Design review of the part shown in the three views and the two pictorial views. Dimensions are in mm from the part's minimum x, y and z. A direction names the side the tool comes from. Round coordinates to 2 decimals unless told otherwise and drop trailing zeros. Loops run counter-clockwise (first coordinate to the right, second up) from the corner with the lowest first, then second, coordinate; pieces in that order, holes last.
1. Consider section B-B on z = 15. State the section outline as (x, y) points.
2. Consider section D-D on y = 23. State the section outline as (x, z) points, then the cut area to 3 significant figures.
3. Tool access review of the marked faces 1 and 2: name each direction out of +Z, -Z, +X, -X, +Y, -Y from which nothing blocks a thin tool from reaching the whole face with its end or side.
4. Clearance check with flat-ended pins moving along their axes: pin 1 Ø10 at (x, z) = (15.5, 9.5) entering from -Y; pin 2 Ø10 at (y, z) = (31.5, 36) entering from +X; pin 3 Ø0.6 at (x, z) = (32.5, 0.5) entering from +Y; pin 4 Ø1 at (x, y) = (26, 0.5) entering from -Z. State where each tip first meets the part, or that it passes through.
5. Consider section C-C on y = 14. State the section outline as (x, z) points.
6. To check wall thickness, follow line 1 along Y through (x, z) = (31.5, 31.5); line 2 along Z through (x, y) = (20, 17); line 3 along X through (y, z) = (41.5, 30.5). State the ranges of each line that lie inside material, in increasing order.
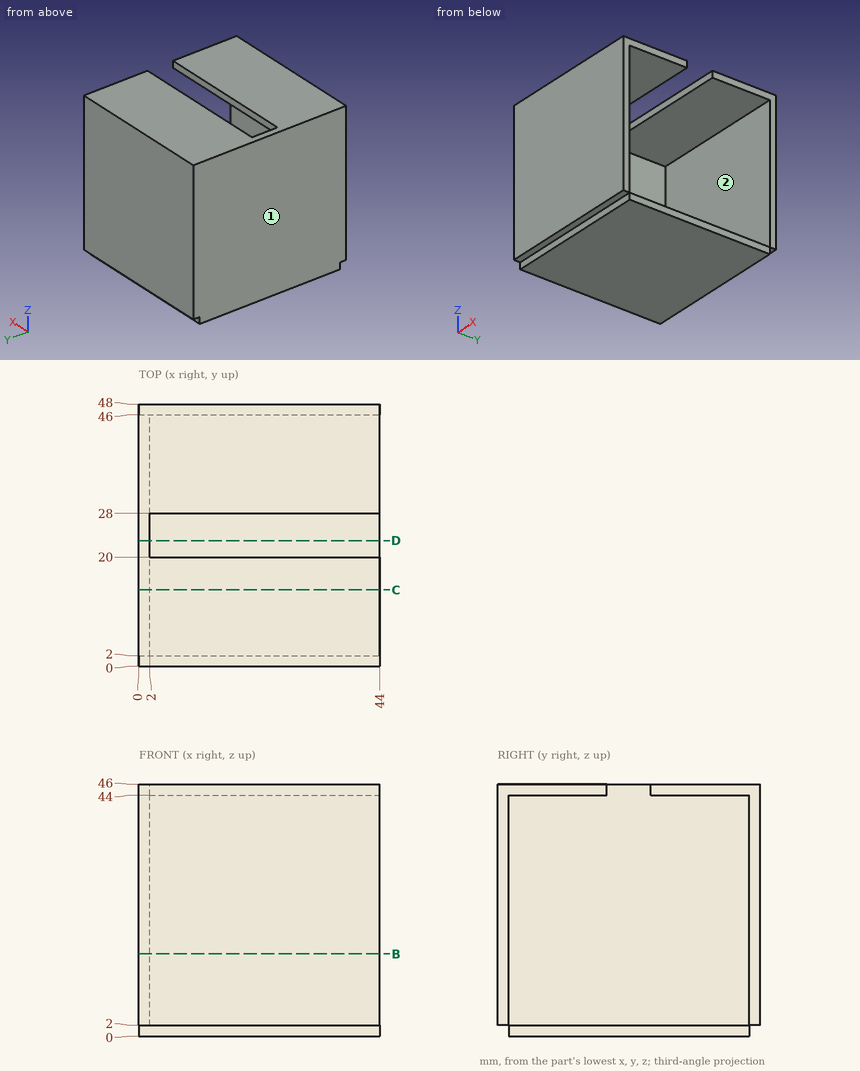
Resolved:
1. outline: (0, 0) - (44, 0) - (44, 2) - (2, 2) - (2, 46) - (44, 46) - (44, 48) - (0, 48) - close
2. outline: (0, 0) - (44, 0) - (44, 2) - (2, 2) - (2, 46) - (0, 46) - close
2. area: 176 mm2
3. face 1: +Z, -Z, -X, +Y, -Y
3. face 2: +X
4. pin 1: stops at y = 0
4. pin 2: stops at x = 2
4. pin 3: stops at y = 46
4. pin 4: stops at z = 2
5. outline: (0, 0) - (44, 0) - (44, 2) - (2, 2) - (2, 44) - (44, 44) - (44, 46) - (0, 46) - close
6. line 1: y = 0 to 2, 46 to 48
6. line 2: z = 0 to 2, 44 to 46
6. line 3: x = 0 to 2
